Part model, mm, in its own coordinate system. Face numbers are marked on the shaded views. A direction names the side the tool comes from. Give positions to 0.01 mm unless a question says otherwise; leave off trailing zeros. Order: outer loops, then holes, each group sorted by start corner. A loop starts at its lowest first (then second) coordinate and runs counter-clockwise, first axis right, second up. Notation, with made-up numbers: (-40, 9) - (-3, 9) arc R27 ccw to (-3, 25) - close; hole circle Ø10 at (-0.5, 46.25). An arc over 180 degrees is marked (long way). Use one line per item in the form item = value. Start each with the question number.
1. Drill centre lines: line 1 (Z direction, x = 0, y = -8.5); line 2 (X direction, y = -47, z = -8); line 3 (Y direction, x = 155, z = -7) (3 decimals). Where is each one in solid material? Low to high.
2. Band-saw the part on B-B, the plane y = -10.5. List the corners of the cut face in (x, z).
3. Tool access for the marked faces 1, 2, 3 and 4: list every direction of +Z, -Z, +X, -X, +Y, -Y with a clear straight run to the whole face (end or side of a thin tool).
4. Band-saw the part on D-D, the plane x = 157.5. List the corners of the cut face in (y, z) (3 decimals), plus the area to 3 significant figures.
5. Pull direction X, two halves, no side cores. Call the marked faces 5, 6 and 7: +X half, -X half, draft (parallel to the pull), parting line (faces both ways), or undercut.
6. Band-saw the part on A-A, the plane x = -7.5. List the corners of the cut face in (y, z) (3 decimals), plus the area to 3 significant figures.
7. Pin check, flat tips, straight feed: P1, Ø3, axis at x = 107.5, y = -13.5, coming from the +Z side; P2, Ø5, axis at y = -48, z = 7, coming from the +X side; P3, Ø1, axis at y = -39.5, z = -1, coming from the -X side. Stop position of each tip, or through.
8. Band-saw the part on C-C, the plane z = 6.5. List the corners of the cut face in (x, y) (3 decimals), plus the area to 3 significant figures.
from build123d import *

# Parameters (mm, degrees)
F0_R     = 12.7
F1_DEPTH = 60.325
F3_DEPTH = 19.05
F4_W     = 46.6944214423
F4_H     = 22.3266
F5_DEPTH = 127
F7_DEPTH = 254
F9_DEPTH = 41.275


with BuildPart() as f1:
    # F0 (on Front) → F1 (new body)
    with BuildSketch(Plane.XZ):
        with BuildLine():
            Line((117.2464, 0), (22.352, 0))
            ThreePointArc((22.352, 0), (-15.8052507731, 15.8052507731), (0, -22.352))
            Line((0, -22.352), (194.2084, -22.352))
            Line((194.2084, -22.352), (194.2084, -7.874))
            ThreePointArc((194.2084, -7.874), (191.9021587951, -2.3062412049), (186.3344, 0))
            Line((186.3344, 0), (150.0886, 0))
            Line((150.0886, 0), (150.0886, 29.718))
            ThreePointArc((150.0886, 29.718), (148.6007024484, 33.3101024484), (145.0086, 34.798))
            Line((145.0086, 34.798), (131.0386, 34.798))
            ThreePointArc((131.0386, 34.798), (127.4644153616, 16.0823576341), (117.2464, 0))
        make_face()
        Circle(F0_R, mode=Mode.SUBTRACT)
    extrude(amount=F1_DEPTH)

    # F2 (on face) → F3 (cut)
    with BuildSketch(Plane.XZ.offset(60.325)):
        Polygon((91.8464, -22.352), (117.2464, -22.352), (117.2464, 0), (85.852, 0), align=None)
    extrude(amount=-F3_DEPTH, mode=Mode.SUBTRACT)

    # F4 (on Top) → F5 (cut, symmetric)
    with BuildSketch(Plane.XY):
        with Locations((0.9952107211, -30.1625)):
            Rectangle(F4_W, F4_H)
    extrude(amount=F5_DEPTH, both=True, mode=Mode.SUBTRACT)

    # F6 (on Top) → F7 (cut)
    with BuildSketch(Plane.XY):
        with BuildLine():
            ThreePointArc((155.3464, -16.002), (150.8562719395, -26.8421280605), (161.6964, -22.352))
            ThreePointArc((161.6964, -22.352), (159.8365280605, -17.8618719395), (155.3464, -16.002))
        make_face()
    extrude(amount=-F7_DEPTH, mode=Mode.SUBTRACT)

    # F8 (on face) → F9 (cut)
    with BuildSketch(Plane(origin=(0, 0, 0), x_dir=(-1, 0, 0), z_dir=(0, 1, 0))):
        with BuildLine():
            Line((-150.0886, 29.718), (-150.0886, 0))
            Line((-150.0886, 0), (-117.2464, 0))
            ThreePointArc((-117.2464, 0), (-127.4644153616, 16.0823576341), (-131.0386, 34.798))
            Line((-131.0386, 34.798), (-145.0086, 34.798))
            ThreePointArc((-145.0086, 34.798), (-148.6007024484, 33.3101024484), (-150.0886, 29.718))
        make_face()
    extrude(amount=-F9_DEPTH, mode=Mode.SUBTRACT)


solid = f1.part
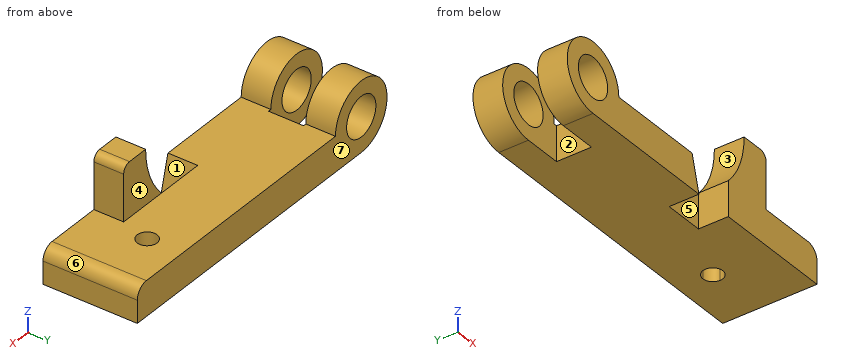
From the geometry:
q1.line_1 = -22.35 to -12.7, 12.7 to 22.35
q1.line_2 = -20.87 to -9.86, 9.86 to 88, 117.25 to 194.21
q1.line_3 = -60.325 to -28.693, -16.011 to 0
q2.outline = (0, -22.35) - (194.21, -22.35) - (194.21, -7.87) arc R7.87 ccw to (186.33, 0) - (22.35, 0) arc R22.35 ccw (long way) to start; hole circle Ø25.4 at (0, 0)
q3.face_1 = +Z, -Y
q3.face_2 = +Z, -Z, -X
q3.face_3 = +Z, +Y, -Y
q3.face_4 = +Z, +X, -X, +Y
q4.outline = (-60.325, -22.352) - (-28.326, -22.352) - (-28.326, 0) - (-60.325, 0) - close; (-16.378, -22.352) - (0, -22.352) - (0, 0) - (-16.378, 0) - close
q4.area = 1,080 mm²
q5.face_5 = undercut
q5.face_6 = +X half
q5.face_7 = draft
q6.outline = (-60.325, -21.056) - (-41.326, -21.056) - (-41.326, -10.249) - (-60.325, -10.249) - close; (-60.325, 10.249) - (-41.326, 10.249) - (-41.326, 21.056) - (-60.325, 21.056) - close; (-18.999, -21.056) - (0, -21.056) - (0, -10.249) - (-18.999, -10.249) - close; (-18.999, 10.249) - (0, 10.249) - (0, 21.056) - (-18.999, 21.056) - close
q6.area = 821 mm²
q7.P1 = 0
q7.P2 = 150.09
q7.P3 = 24.34
q8.outline = (-21.386, -60.325) - (-10.911, -60.325) - (-10.911, -41.326) - (-21.386, -41.326) - close; (-21.386, -18.999) - (-10.911, -18.999) - (-10.911, 0) - (-21.386, 0) - close; (10.911, -60.325) - (21.386, -60.325) - (21.386, -41.326) - (10.911, -41.326) - close; (10.911, -18.999) - (21.386, -18.999) - (21.386, 0) - (10.911, 0) - close; (122.425, -60.325) - (150.089, -60.325) - (150.089, -41.275) - (122.425, -41.275) - close
q8.area = 1,320 mm²
